```python
from build123d import *

# Parameters (mm, degrees)
SKETCH1_R               = 12.5
BOSS_EXTRUDE4_DEPTH     = 3
CUT_EXTRUDE_THIN3_START = -3
CUT_EXTRUDE_THIN3_DEPTH = 3


# Read off the part's stored shape, not the designer's step: Cut-Extrude-Thin3
with BuildPart() as part:
    # Sketch1 → Boss-Extrude4 (new body)
    with BuildSketch(Plane.XY):
        Polygon((-40, 47), (40, 47), (47, 47), (47, 40), (47, -40), (47, -47), (40, -47), (-40, -47), (-47, -47), (-47, -40), (-47, 40), (-47, 47), align=None)
        Circle(SKETCH1_R, mode=Mode.SUBTRACT)
        with BuildLine():
            Line((-27.5, 32.5), (27.5, 32.5))
            Line((27.5, 32.5), (9.624571705, 14.615663498))
            ThreePointArc((9.624571705, 14.615663498), (0.00658569, 17.499998761), (-9.613568497, 14.622903294))
            Line((-9.613568497, 14.622903294), (-27.5, 32.5))
        make_face(mode=Mode.SUBTRACT)
        with BuildLine():
            Line((-32.5, 27.5), (-32.5, -27.529900959))
            Line((-32.5, -27.529900959), (-14.610866481, -9.631852402))
            ThreePointArc((-14.610866481, -9.631852402), (-17.49999836, -0.007575188), (-14.619199644, 9.619199644))
            Line((-14.619199644, 9.619199644), (-32.5, 27.5))
        make_face(mode=Mode.SUBTRACT)
        with BuildLine():
            Line((-27.5, -32.5), (27.5, -32.5))
            Line((27.5, -32.5), (9.619199644, -14.619199644))
            ThreePointArc((9.619199644, -14.619199644), (0, -17.5), (-9.619199644, -14.619199644))
            Line((-9.619199644, -14.619199644), (-27.5, -32.5))
        make_face(mode=Mode.SUBTRACT)
        with BuildLine():
            Line((32.5, 27.5), (14.619199644, 9.619199644))
            ThreePointArc((14.619199644, 9.619199644), (17.4999982, 0.007937724), (14.627919862, -9.60593361))
            Line((14.627919862, -9.60593361), (32.5, -27.5))
            Line((32.5, -27.5), (32.5, 27.5))
        make_face(mode=Mode.SUBTRACT)
    extrude(amount=BOSS_EXTRUDE4_DEPTH)

    # Cut-Extrude-Thin3 outline → Cut-Extrude-Thin3 (cut)
    with BuildSketch(Plane(origin=(0, 0, 0), x_dir=(-1, 0, 0), z_dir=(0, 0, -1)).offset(CUT_EXTRUDE_THIN3_START)):
        Polygon((-42, -41), (-42, -32), (-47, -32), (-47, -47), (-39.999705668, -47), (-39.999705668, -44), (-34.999705668, -44), (-34.999705668, -41), align=None)
        Polygon((-47, 47), (-47, 32), (-42, 32), (-42, 41), (-34.999705668, 41), (-34.999705668, 44), (-39.999705668, 44), (-39.999705668, 47), align=None)
        Polygon((0, -46.846551451), (-39.999705668, -47), (39.999705668, -47), align=None)
        Polygon((39.999705668, -44), (39.999705668, -47), (47, -47), (47, -32), (42, -32), (42, -41), (34.999705668, -41), (34.999705668, -44), align=None)
        Polygon((39.999705668, 47), (-39.999705668, 47), (0, 46.846551451), align=None)
        Polygon((47, 47), (39.999705668, 47), (39.999705668, 44), (34.999705668, 44), (34.999705668, 41), (42, 41), (42, 32), (47, 32), align=None)
    extrude(amount=CUT_EXTRUDE_THIN3_DEPTH, mode=Mode.SUBTRACT)


solid = part.part
```
Can you work these out from the model? Positions are in its coordinate system, mm. A direction names the side the tool comes from. Coordinates: 2 decimals unless noted, no trailing zeros. Loops run counter-clockwise (first coordinate to the right, second up) from the corner with the lowest first, then second, coordinate; pieces in that order, holes last. Notation, with made-up numbers: (60, 29) -> (73, 29) arc R11 cw to (73, 37) -> close; hole circle Ø8 at (77, 17.5). An arc over 180 degrees is marked (long way). Put each result on its own line as item: value. Start each with the question number.
Q1. If I drill on line 1 (X direction, y = -0.5, z = 0.95); line 2 (Y direction, x = -39, z = 1.75); line 3 (Y direction, x = 0, z = 1.2), over which ranges is the centre line in solid material (lowest first)? Write a range as [from, to].
Q2. For faces 4 (the face through (-40, -45, 2)), 5 (the face through (45, 32, 2)), 6 (the face through (44, -32, 2)), which set-ups out of +Z, -Z, +X, -X, +Y, -Y let a thin tool reach every point of the face, with its end or its side?
Q3. I want a section at C-C (z = 1.4). Count the separate pieces of the cut face and the enclosed holes in it, plus the area to 3 significant figures.
Q4. I want a section at A-A (y = 0). Write out the boundary of the cut face in (x, z), plus the area to 3 significant figures.
Q5. Thinking about a two-plate mould opening in X: for faces 1 (the face through (-39, -41, 2)), 2 (the face through (-17.5, -0.2, 1.5)), 3 (the face through (35, -43, 2)), which applies, pulls with the +X half, pulls with the -X half, needs draft (parallel to the pull), parting line crosses it, or undercut?
Q6. I'm going to push flat-ended pins straight in: P1, Ø0.9, axis at y = -43, z = 1, coming from the +X side; P2, Ø1.5, axis at y = 42, z = 2, coming from the -X side; P3, Ø0.9, axis at x = 39, z = 1, coming from the -Y side; P4, Ø1, axis at x = -8.5, y = -16, coming from the +Z side. Where does each tip first touch, or does it pass through?
Q7. I want a section at B-B (x = -23). Write out the boundary of the cut face in (y, z).
Taken from the geometry:
1. line 1: x = [-47, -32.5], [-17.49, -12.49], [12.49, 17.49], [32.5, 47]
1. line 2: y = [-47, -44], [-41, 41], [44, 47]
1. line 3: y = [-46.85, -32.5], [-17.5, -12.5], [12.5, 17.5], [32.5, 46.85]
2. face 4: +Z, -Z, -X, -Y
2. face 5: +Z, -Z, +X, +Y
2. face 6: +Z, -Z, +X, -Y
3. separate pieces: 1
3. enclosed holes: 5
3. area: 5,420 mm2
4. outline: (-47, 0) -> (-32.5, 0) -> (-32.5, 3) -> (-47, 3) -> close; (-17.5, 0) -> (-12.5, 0) -> (-12.5, 3) -> (-17.5, 3) -> close; (12.5, 0) -> (17.5, 0) -> (17.5, 3) -> (12.5, 3) -> close; (32.5, 0) -> (47, 0) -> (47, 3) -> (32.5, 3) -> close
4. area: 117 mm2
5. face 1: needs draft
5. face 2: undercut
5. face 3: pulls with the +X half
6. P1: stops at x = 35
6. P2: stops at x = -35
6. P3: stops at y = -47
6. P4: passes through
7. outline: (-46.93, 0) -> (-32.5, 0) -> (-32.5, 3) -> (-46.93, 3) -> close; (-28, 0) -> (-18.03, 0) -> (-18.03, 3) -> (-28, 3) -> close; (18, 0) -> (28, 0) -> (28, 3) -> (18, 3) -> close; (32.5, 0) -> (46.93, 0) -> (46.93, 3) -> (32.5, 3) -> close
